Input: part model. Units: mm. Frame: model coordinates. A direction names the side the tool comes from. Give positions to 0.01 mm unless a question says otherwise; leave off trailing zeros. Loops run counter-clockwise (first coordinate to the right, second up) from the corner with the lowest first, then second, coordinate; pieces in that order, holes last. Notation, with made-up numbers: (69, -1) -> (94, -1) arc R25 ccw to (94, 25) -> close; hole circle Ø6 at (18, 44.25). An arc over 180 degrees is marked (long way). Answer in a Markdown table with one row per item. Add a question column.
```python
from build123d import *

# Parameters (mm, degrees)
BOSS_EXTRUDE1_DEPTH = 6
SKETCH2_W           = 10
SKETCH2_H           = 6
BOSS_EXTRUDE2_DEPTH = 6
SKETCH3_W           = 10
SKETCH3_H           = 6
BOSS_EXTRUDE3_DEPTH = 6
SKETCH4_W           = 20
SKETCH4_H           = 30.367424907
CUT_EXTRUDE1_DEPTH  = 6
CUT_EXTRUDE2_DEPTH  = 355.990492973
FLEX1_DEPTH         = 6
FLEX1_2_DEPTH       = 6


# Read off the part's stored shape, not the designer's step: Flex1
with BuildPart() as part:
    # Sketch1 → Boss-Extrude1 (new body)
    with BuildSketch(Plane(origin=(0, 0, 0), x_dir=(1, 0, 0), z_dir=(0, 1, 0))):
        with BuildLine():
            Line((0, 0), (0, 66.5))
            add(Edge.make_bspline(
                [(0, 66.5), (0, 168.087947667), (114.415275211, 225.5), (260, 225.5)],
                knots=[0, 0, 0, 0, 1, 1, 1, 1], degree=3))
            Line((260, 225.5), (260, 255.5))
            Line((260, 255.5), (0, 255.5))
            add(Edge.make_bspline(
                [(-80, 66.5), (-80, 138.367791909), (0, 189.401588521), (0, 255.5)],
                knots=[0, 0, 0, 0, 1, 1, 1, 1], degree=3))
            Line((-80, 66.5), (-80, 0))
            Line((-80, 0), (0, 0))
        make_face()
    extrude(amount=BOSS_EXTRUDE1_DEPTH)

    # Sketch2 → Boss-Extrude2 (add)
    with BuildSketch(Plane(origin=(0, 6, 0), x_dir=(1, 0, 0), z_dir=(0, 1, 0))):
        with Locations((-35, -3)):
            Rectangle(SKETCH2_W, SKETCH2_H)
        with Locations((-15, -3)):
            Rectangle(SKETCH2_W, SKETCH2_H)
        with Locations((-55, -3)):
            Rectangle(SKETCH2_W, SKETCH2_H)
        with Locations((-75, -3)):
            Rectangle(SKETCH2_W, SKETCH2_H)
    extrude(amount=-BOSS_EXTRUDE2_DEPTH)

    # Sketch3 → Boss-Extrude3 (add)
    with BuildSketch(Plane(origin=(0, 6, 0), x_dir=(1, 0, 0), z_dir=(0, 1, 0))):
        with Locations((195, 258.5)):
            Rectangle(SKETCH3_W, SKETCH3_H)
        with Locations((225, 258.5)):
            Rectangle(SKETCH3_W, SKETCH3_H)
        with Locations((165, 258.5)):
            Rectangle(SKETCH3_W, SKETCH3_H)
        with Locations((135, 258.5)):
            Rectangle(SKETCH3_W, SKETCH3_H)
        with Locations((105, 258.5)):
            Rectangle(SKETCH3_W, SKETCH3_H)
        with Locations((75, 258.5)):
            Rectangle(SKETCH3_W, SKETCH3_H)
        with Locations((45, 258.5)):
            Rectangle(SKETCH3_W, SKETCH3_H)
        with Locations((15, 258.5)):
            Rectangle(SKETCH3_W, SKETCH3_H)
    extrude(amount=-BOSS_EXTRUDE3_DEPTH)

    # Sketch4 → Cut-Extrude1 (cut)
    with BuildSketch(Plane(origin=(0, 6, 0), x_dir=(1, 0, 0), z_dir=(0, 1, 0))):
        with Locations((250, 240.316287547)):
            Rectangle(SKETCH4_W, SKETCH4_H)
    extrude(amount=-CUT_EXTRUDE1_DEPTH, mode=Mode.SUBTRACT)

    # Sketch5 → Cut-Extrude2 (cut, through all)
    with BuildSketch(Plane(origin=(0, 6, 0), x_dir=(1, 0, 0), z_dir=(0, 1, 0))):
        Polygon((-29.891687561, 144.39007032), (-34.642769417, 147.71681365), (-23.285955978, 163.936024127), (-18.534874121, 160.609280796), align=None)
        Polygon((-58.550195169, 103.425626242), (-63.308179345, 106.742490211), (-51.985092004, 122.985263776), (-47.227107828, 119.668399807), align=None)
    extrude(amount=-CUT_EXTRUDE2_DEPTH, mode=Mode.SUBTRACT)

    # Flex1 outline → Flex1 (cut)
    with BuildSketch(Plane(origin=(0, 0, 0), x_dir=(1, 0, 0), z_dir=(0, 1, 0))):
        with BuildLine():
            add(Edge.make_bspline(
                [(0, 90.229900389), (0, 187.117415556), (104.072328665, 243.822461296), (240.00000001, 248.862475483)],
                knots=[0, 0, 0, 0, 0.953730412, 0.953730412, 0.953730412, 0.953730412], degree=3))
            Line((0, 90.229900389), (0, 66.5))
            add(Edge.make_bspline(
                [(0, 66.5), (0, 163.387515167), (104.072328665, 220.092560907), (240.00000001, 225.132575093)],
                knots=[0, 0, 0, 0, 0.953730412, 0.953730412, 0.953730412, 0.953730412], degree=3))
            Line((240.00000001, 225.132575093), (240.00000001, 248.862475483))
        make_face()
        with BuildLine():
            add(Edge.make_bspline(
                [(-51.148803226, 146.132174392), (-54.710438553, 140.513781755), (-58.143911828, 134.842056067), (-61.323392575, 129.088765208)],
                knots=[0.594014657, 0.594014657, 0.594014657, 0.594014657, 0.686318961, 0.686318961, 0.686318961, 0.686318961], degree=3))
            Line((-61.323392575, 129.088765208), (-58.550195169, 127.155526632))
            Line((-58.550195169, 127.155526632), (-47.227107828, 143.398300196))
            Line((-47.227107828, 143.398300196), (-51.148803226, 146.132174392))
        make_face()
        with BuildLine():
            add(Edge.make_bspline(
                [(-31.878447999, 175.394574164), (-32.758957733, 174.05373382), (-33.644948776, 172.71267215), (-34.534615872, 171.370984112)],
                knots=[0.431899292, 0.431899292, 0.431899292, 0.431899292, 0.454328108, 0.454328108, 0.454328108, 0.454328108], degree=3))
            Line((-34.534615872, 171.370984112), (-29.891687561, 168.119970709))
            Line((-29.891687561, 168.119970709), (-18.534874121, 184.339181186))
            Line((-18.534874121, 184.339181186), (-23.285955978, 187.665924517))
            Line((-23.285955978, 187.665924517), (-31.878447999, 175.394574164))
        make_face()
    extrude(amount=FLEX1_DEPTH, mode=Mode.SUBTRACT)

    # Flex1 2 outline → Flex1 2 (add)
    with BuildSketch(Plane(origin=(0, 0, 0), x_dir=(1, 0, 0), z_dir=(0, 1, 0))):
        with BuildLine():
            Line((230, 255.5), (240, 255.5))
            Line((240, 255.5), (240, 279.229900389))
            Line((240, 279.229900389), (230, 279.229900389))
            Line((230, 279.229900389), (230, 285.229900389))
            Line((230, 285.229900389), (220, 285.229900389))
            Line((220, 285.229900389), (220, 279.229900389))
            Line((220, 279.229900389), (200, 279.229900389))
            Line((200, 279.229900389), (200, 285.229900389))
            Line((200, 285.229900389), (190, 285.229900389))
            Line((190, 285.229900389), (190, 279.229900389))
            Line((190, 279.229900389), (170, 279.229900389))
            Line((170, 279.229900389), (170, 285.229900389))
            Line((170, 285.229900389), (160, 285.229900389))
            Line((160, 285.229900389), (160, 279.229900389))
            Line((160, 279.229900389), (140, 279.229900389))
            Line((140, 279.229900389), (140, 285.229900389))
            Line((140, 285.229900389), (130, 285.229900389))
            Line((130, 285.229900389), (130, 279.229900389))
            Line((130, 279.229900389), (110, 279.229900389))
            Line((110, 279.229900389), (110, 285.229900389))
            Line((110, 285.229900389), (100, 285.229900389))
            Line((100, 285.229900389), (100, 279.229900389))
            Line((100, 279.229900389), (80, 279.229900389))
            Line((80, 279.229900389), (80, 285.229900389))
            Line((80, 285.229900389), (70, 285.229900389))
            Line((70, 285.229900389), (70, 279.229900389))
            Line((70, 279.229900389), (50, 279.229900389))
            Line((50, 279.229900389), (50, 285.229900389))
            Line((50, 285.229900389), (40, 285.229900389))
            Line((40, 285.229900389), (40, 279.229900389))
            Line((40, 279.229900389), (20, 279.229900389))
            Line((20, 279.229900389), (20, 285.229900389))
            Line((20, 285.229900389), (10, 285.229900389))
            Line((10, 285.229900389), (10, 279.229900389))
            Line((10, 279.229900389), (0, 279.229900389))
            add(Edge.make_bspline(
                [(0, 279.229900389), (0, 213.131488911), (-80, 162.097692299), (-80, 90.229900389)],
                knots=[0, 0, 0, 0, 1, 1, 1, 1], degree=3))
            Line((-80, 90.229900389), (-80, 66.5))
            add(Edge.make_bspline(
                [(-61.323392575, 129.088765208), (-72.12833646, 109.537149765), (-80, 89.04356364), (-80, 66.5)],
                knots=[0.686318961, 0.686318961, 0.686318961, 0.686318961, 1, 1, 1, 1], degree=3))
            Line((-61.323392575, 129.088765208), (-63.308179345, 130.4723906))
            Line((-63.308179345, 130.4723906), (-51.985092004, 146.715164165))
            Line((-51.985092004, 146.715164165), (-51.148803226, 146.132174392))
            add(Edge.make_bspline(
                [(-34.534615872, 171.370984112), (-40.075457788, 163.01495819), (-45.758886122, 154.634636824), (-51.148803226, 146.132174392)],
                knots=[0.454328108, 0.454328108, 0.454328108, 0.454328108, 0.594014657, 0.594014657, 0.594014657, 0.594014657], degree=3))
            Line((-34.534615872, 171.370984112), (-34.642769417, 171.44671404))
            Line((-34.642769417, 171.44671404), (-31.878447999, 175.394574164))
            add(Edge.make_bspline(
                [(0, 255.5), (0, 226.952142889), (-14.922959865, 201.214393816), (-31.878447999, 175.394574164)],
                knots=[0, 0, 0, 0, 0.431899292, 0.431899292, 0.431899292, 0.431899292], degree=3))
            Line((0, 255.5), (10, 255.5))
            Line((10, 255.5), (10, 261.5))
            Line((10, 261.5), (20, 261.5))
            Line((20, 261.5), (20, 255.5))
            Line((20, 255.5), (40, 255.5))
            Line((40, 255.5), (40, 261.5))
            Line((40, 261.5), (50, 261.5))
            Line((50, 261.5), (50, 255.5))
            Line((50, 255.5), (70, 255.5))
            Line((70, 255.5), (70, 261.5))
            Line((70, 261.5), (80, 261.5))
            Line((80, 261.5), (80, 255.5))
            Line((80, 255.5), (100, 255.5))
            Line((100, 255.5), (100, 261.5))
            Line((100, 261.5), (110, 261.5))
            Line((110, 261.5), (110, 255.5))
            Line((110, 255.5), (130, 255.5))
            Line((130, 255.5), (130, 261.5))
            Line((130, 261.5), (140, 261.5))
            Line((140, 261.5), (140, 255.5))
            Line((140, 255.5), (160, 255.5))
            Line((160, 255.5), (160, 261.5))
            Line((160, 261.5), (170, 261.5))
            Line((170, 261.5), (170, 255.5))
            Line((170, 255.5), (190, 255.5))
            Line((190, 255.5), (190, 261.5))
            Line((190, 261.5), (200, 261.5))
            Line((200, 261.5), (200, 255.5))
            Line((200, 255.5), (220, 255.5))
            Line((220, 255.5), (220, 261.5))
            Line((220, 261.5), (230, 261.5))
            Line((230, 261.5), (230, 255.5))
        make_face()
        Polygon((0, -9.270099611), (0, 0), (-10, 0), (-10, -6), (-20, -6), (-20, 0), (-30, 0), (-30, -6), (-40, -6), (-40, 0), (-50, 0), (-50, -6), (-60, -6), (-60, 0), (-70, 0), (-70, -6), (-80, -6), (-80, -15.270099611), (-70, -15.270099611), (-70, -9.270099611), (-60, -9.270099611), (-60, -15.270099611), (-50, -15.270099611), (-50, -9.270099611), (-40, -9.270099611), (-40, -15.270099611), (-30, -15.270099611), (-30, -9.270099611), (-20, -9.270099611), (-20, -15.270099611), (-10, -15.270099611), (-10, -9.270099611), align=None)
        Polygon((-63.308179345, 106.742490211), (-58.550195169, 103.425626242), (-47.227107828, 119.668399807), (-51.985092004, 122.985263776), align=None)
        Polygon((-34.642769417, 147.71681365), (-29.891687561, 144.39007032), (-18.534874121, 160.609280796), (-23.285955978, 163.936024127), align=None)
    extrude(amount=FLEX1_2_DEPTH)


solid = part.part
```
1) Reachability of faces 1 (the face through (-57.726, 2.958, -138.48)), 2 (the face through (20, 6, -169)) from +Z, -Z, +X, -X, +Y, -Y: full face, straight path, thin tool, end or side. Return the list, or none.
2) Material intervals for line 1 along X through (y, z) = (2.25, -27.5); line 2 along Z through (x, y) = (-32, 3.5); line 3 along X through (y, z) = (2, -170), sorted ascending.
3) Pin query (flat end, axial travel): pin 1 (1.8 mm diameter, centred on y = 1.5, z = -281.5, fed in from +X); pin 2 (3 mm diameter, centred on x = -43.5, y = 4, fed in from +Z); pin 3 (3 mm diameter, centred on x = 147.5, y = 3.5, fed in from -Z). Return the tip coordinate at first contact, or that it passes through.
4) Section B-B on z = -7. Output: boundary loops of the cut face in (x, y).
5) Pull-direction query (Z, two-part tool) for faces 3 (the face through (20, 0, -169)), 4 (the face through (-52.97, 2.96, -135.16)), 5 (the face through (-24.29, 2.96, -176.12)); classes: +Z half, -Z half, draft (parallel to the pull), parting line (faces both ways), or undercut.
6) Section A-A on y = 3. State how many separate pieces and enclosed holes the cut face has, and give its area (3 significant figures).
Working result:
| question | item | result |
|---|---|---|
| 1 | face 1 | +Y, -Y |
| 1 | face 2 | +Z, -Z, +X, -X, +Y |
| 2 | line 1 | x = -80 to 0 |
| 2 | line 2 | z = -198.94 to -175.22, -169.6 to 15.27 |
| 2 | line 3 | x = -51.06 to -32.58, -28.58 to 29.17 |
| 3 | pin 1 | stops at x = 230 |
| 3 | pin 2 | stops at z = 9.27 |
| 3 | pin 3 | stops at z = -279.23 |
| 4 | outline | (-80, 0) -> (0, 0) -> (0, 6) -> (-80, 6) -> close |
| 5 | face 3 | draft |
| 5 | face 4 | undercut |
| 5 | face 5 | undercut |
| 6 | separate pieces | 1 |
| 6 | enclosed holes | 2 |
| 6 | area | 31,400 mm2 |
